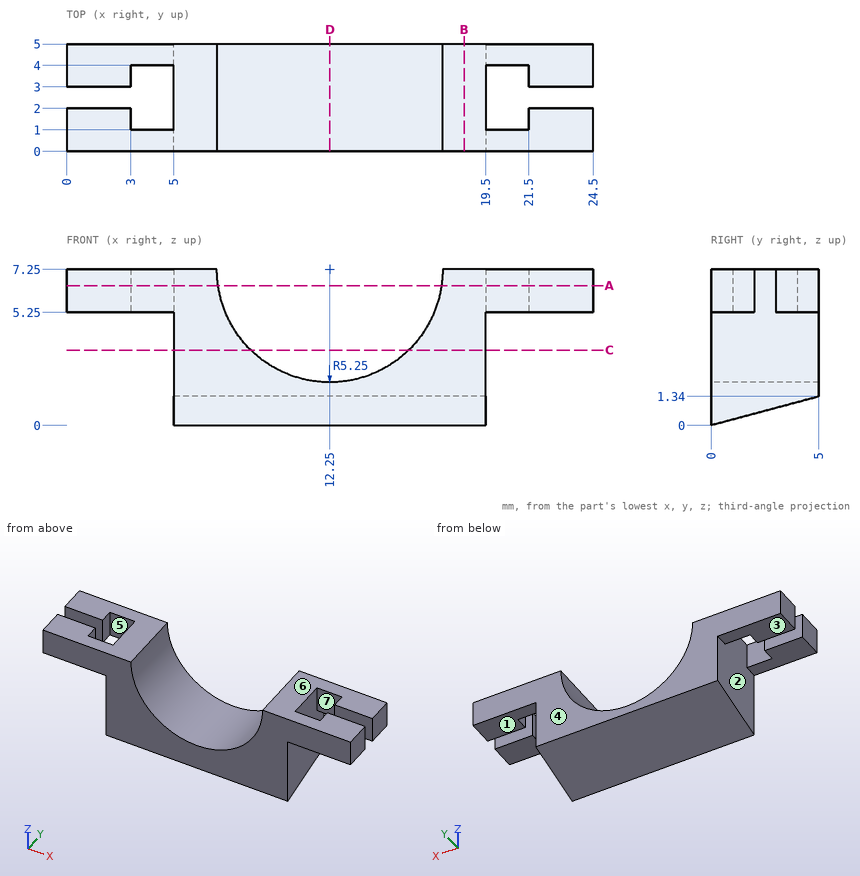
The drawing under review shows one solid part. Ordinate dimensions are in mm from its lowest x, y, z. A direction names the side the tool comes from. Round coordinates to 2 decimals unless told otherwise and drop trailing zeros. Write each loop counter-clockwise with the first axis right and the second up, starting at its lowest first coordinate (ties: lowest second). Pieces come first, ordered by that corner, then holes. Notation, with made-up numbers: (88, 39.25) - (127, 39.25) arc R12 cw to (127, 58.25) - close; hole circle Ø11 at (42.5, 76). An arc over 180 degrees is marked (long way). Put each result on its own line as item: value.
Q1. Wall thickness on probe 1 along Y at (x, z) = (22, 7); probe 2 along X at (y, z) = (3.15, 7); probe 3 along X at (y, z) = (1.1, 6): over which ranges is each line inside the solid? List them lowest first.
Solved:
probe 1: y = 0 to 2, 3 to 5
probe 2: x = 0 to 3, 5 to 7.01, 17.49 to 19.5, 21.5 to 24.5
probe 3: x = 0 to 3, 5 to 7.15, 17.35 to 19.5, 21.5 to 24.5
Q2. Insertion check: pin 1 Ø1.6 at (x, y) = (22.5, 1) entering from -Z; pin 2 Ø1 at (x, y) = (12.5, 1) entering from +Z. Each pin has a flat end and moves straight along its axis. Give the tip position at first contact, or say it passes through.
Solved:
pin 1: stops at z = 5.25
pin 2: stops at z = 2.05
Q3. We need section A-A (z = 6.5). Give the boundary of the cut face in (x, y).
Solved:
outline: (0, 0) - (7.05, 0) - (7.05, 5) - (0, 5) - (0, 3) - (3, 3) - (3, 4) - (5, 4) - (5, 1) - (3, 1) - (3, 2) - (0, 2) - close; (17.45, 0) - (24.5, 0) - (24.5, 2) - (21.5, 2) - (21.5, 1) - (19.5, 1) - (19.5, 4) - (21.5, 4) - (21.5, 3) - (24.5, 3) - (24.5, 5) - (17.45, 5) - close
Q4. Mouldability with a two-part tool opening along Y and no side actions: class the marked faces 4, 5, 6 and 7 as released by +Y, released by -Y, zero draft, split by the parting line, or undercut.
Solved:
face 4: released by +Y
face 5: undercut
face 6: zero draft
face 7: undercut
Q5. We need section D-D (x = 12.25). Give the boundary of the cut face in (y, z).
Solved:
outline: (0, 0) - (5, 1.34) - (5, 2) - (0, 2) - close
Q6. We need section C-C (z = 3.5). Give the boundary of the cut face in (x, y).
Solved:
outline: (5, 0) - (8.58, 0) - (8.58, 5) - (5, 5) - close; (15.92, 0) - (19.5, 0) - (19.5, 5) - (15.92, 5) - close
Q7. We need section B-B (x = 18.5). Give the boundary of the cut face in (y, z), and give its area (3 significant figures).
Solved:
outline: (0, 0) - (5, 1.34) - (5, 7.25) - (0, 7.25) - close
area: 32.9 mm2
Q8. Machinability: for the marked faces 1, 2 and 3, which of the approach directions +Z, -Z, +X, -X, +Y, -Y give a long, thin tool a straight path to every point of the face, cutting with its end or side? Answer none if there is none.
Solved:
face 1: -Z, +X, +Y, -Y
face 2: -Z
face 3: -Z, -X, +Y, -Y
